Autodesk Inventor part; units mm, degrees
ref_plane "YZ Plane" through (0, 0, 0) normal (1, 0, 0) x (0, 1, 0)
ref_plane "XZ Plane" through (0, 0, 0) normal (0, 1, 0) x (-1, 0, 0)
ref_plane "XY Plane" through (0, 0, 0) normal (0, 0, 1) x (1, 0, 0)
sketch "Sketch1" plane through (0, 0, 0) normal (0, 1, 0) x (-1, 0, 0)
  circle A0 centre (0, 0) radius 2.5
  dimension "d0" = 5
extrude "Extrusion1" add sketch "Sketch1" along normal blind 12
sketch "Sketch2" plane through (0, 12, 0) normal (0, 1, 0) x (1, 0, 0)
  circle A0 centre (0, 0) radius 2.5
  circle A1 centre (0, 0) radius 4.25
  dimension "d3" = 8.5
extrude "Extrusion2" add sketch "Sketch2" along normal blind 5 contours A0 | A1
sketch "Sketch3" plane through (0, 17, 0) normal (0, 1, 0) x (1, 0, 0)
  circle A0 centre (0, 0) radius 4.25
  line L0 (0, 2.3094) -> (2, 1.1547)
  line L1 (2, 1.1547) -> (2, -1.1547)
  line L2 (2, -1.1547) -> (0, -2.3094)
  line L3 (0, -2.3094) -> (-2, -1.1547)
  line L4 (-2, -1.1547) -> (-2, 1.1547)
  line L5 (-2, 1.1547) -> (0, 2.3094)
  dimension "d6" = 2
extrude "Extrusion3" cut sketch "Sketch3" against normal blind 3.2 contours L0 L1 L2 L3 L4 L5
thread "Thread1"
chamfer "Chamfer1" distance 0.25 angle 45 1 edges at (2.5, 0, 0)
properties part number "M5x12SHCS" material "Stainless Steel"
Build history of the part. All positions in model axes, mm. A direction names the side the tool comes from. Coordinates: 2 decimals unless noted, no trailing zeros. Write each loop counter-clockwise with the first axis right and the second up, starting at its lowest first coordinate (ties: lowest second). Pieces come first, ordered by that corner, then holes. Notation, with made-up numbers: (-2, 0.5) -> (17, 0.5) arc R16 ccw to (17, 6.5) -> close; hole circle Ø4 at (27, -16.75). An arc over 180 degrees is marked (long way). Use CSV: the item, a comma, the result in double quotes. Start each with the question number.
Q1. Drill centre lines: probe 1 along Y at (x, z) = (-1.25, -3.5); probe 2 along Y at (x, z) = (0, -1.75); probe 3 along X at (y, z) = (1.75, -1.5). Where is each one in solid material? Low to high.
Q2. 3-axis set-ups, long thin cutter, end or side, ignore diameter. For faces 4 (the flat face through (0, 0, 0)), 5 (the flat face through (0, 13.8, 0)), 6 (the flat face through (2, 12, 2)): which of +Z, -Z, +X, -X, +Y, -Y reach the whole face in a straight line?
Q3. Cut at C-C, the plane x = 3.75. List the corners of the cut face in (y, z).
Q4. Cut at A-A, the plane z = 0. List the corners of the cut face in (x, y), then the cut area to 3 significant figures.
Q5. Flat gauge pins, fed straight in: pin 1 Ø3 at (x, y) = (2.5, 6) entering from +Z; pin 2 Ø2 at (x, y) = (1.5, 13) entering from -Z; pin 3 Ø2 at (x, z) = (0, 0.5) entering from +Y. Where does each tip first touch, or does it go through?
Q6. Cut at B-B, the plane y = 6.5. List the corners of the cut face in (x, z).
Q7. Pull direction X, two halves, no side cores. Call faces 1 (the flat face through (2, 15, 0)), 2 (the flat face through (1, 17, 2)), 3 (the cylindrical face through (2.285, 14.465, 3.584)): released by +X, released by -X, zero draft, split by the parting line, or undercut.
Q8. Cut at D-D, the plane z = 3.75. List the corners of the cut face in (x, y), then the cut area to 3 significant figures.
Checked values:
1,probe 1,"y = 12 to 17"
1,probe 2,"y = 0 to 13.8"
1,probe 3,"x = -2 to 2"
2,face 4,"+Z, -Z, +X, -X, -Y"
2,face 5,"+Y"
2,face 6,"-Y"
3,outline,"(12, -2) -> (17, -2) -> (17, 2) -> (12, 2) -> close"
4,outline,"(-4.25, 12) -> (-2.5, 12) -> (-2.5, 0.25) -> (-2.25, 0) -> (2.25, 0) -> (2.5, 0.25) -> (2.5, 12) -> (4.25, 12) -> (4.25, 17) -> (2, 17) -> (2, 13.8) -> (-2, 13.8) -> (-2, 17) -> (-4.25, 17) -> close"
4,area,"89.6 mm²"
5,pin 1,"stops at z = 2.29"
5,pin 2,"stops at z = -4.22"
5,pin 3,"stops at y = 13.8"
6,outline,"circle Ø5 at (0, 0)"
7,face 1,"undercut"
7,face 2,"zero draft"
7,face 3,"split by the parting line"
8,outline,"(-2, 12) -> (2, 12) -> (2, 17) -> (-2, 17) -> close"
8,area,"20.0 mm²"
